from build123d import *

# Parameters (mm, degrees)
SKETCH1_R           = 12.5
SKETCH1_R_2         = 9.5
BOSS_EXTRUDE1_DEPTH = 14
SKETCH2_W           = 64.506168934
SKETCH2_H           = 47.83380527
BOSS_EXTRUDE2_DEPTH = 5
SKETCH3_R           = 7.5
CUT_EXTRUDE1_DEPTH  = 5
FILLET1_R           = 10
SKETCH4_R           = 41.339159207
SKETCH4_R_2         = 22.478966411
CUT_EXTRUDE2_DEPTH  = 10
SKETCH5_W           = 60
SKETCH5_H           = 44.957932822
SKETCH5_R           = 6
BOSS_EXTRUDE3_DEPTH = 5
FILLET2_R           = 5
SKETCH6_R           = 7.5
CUT_EXTRUDE3_DEPTH  = 10.435721216
SKETCH7_R           = 14
SKETCH7_R_2         = 12.5
BOSS_EXTRUDE4_DEPTH = 3.5
SKETCH8_R           = 13.175914581
SKETCH8_R_2         = 11.95
CUT_EXTRUDE4_DEPTH  = 2.5
BOSS_EXTRUDE5_START = -14
SKETCH9_R           = 9.5
SKETCH9_R_2         = 7.5
BOSS_EXTRUDE5_DEPTH = 14
SKETCH11_R          = 1.75
CUT_EXTRUDE5_DEPTH  = 6.2


with BuildPart() as part:
    # Sketch1 → Boss-Extrude1 (new body)
    with BuildSketch(Plane(origin=(0, 0, 0), x_dir=(1, 0, 0), z_dir=(0, 1, 0))):
        with Locations(Location((0, 0, 0), (0, 0, 270))):
            Circle(SKETCH1_R)
        with Locations(Location((0, 0, 0), (0, 0, 270))):
            Circle(SKETCH1_R_2, mode=Mode.SUBTRACT)
    extrude(amount=BOSS_EXTRUDE1_DEPTH)

    # Sketch2 → Boss-Extrude2 (add)
    with BuildSketch(Plane(origin=(0, 0, 0), x_dir=(-1, 0, 0), z_dir=(0, -1, 0))):
        Rectangle(SKETCH2_W, SKETCH2_H)
    extrude(amount=BOSS_EXTRUDE2_DEPTH)

    # Sketch3 → Cut-Extrude1 (cut)
    with BuildSketch(Plane(origin=(0, 0, 0), x_dir=(1, 0, 0), z_dir=(0, 1, 0))):
        with Locations(Location((0, 0, 0), (0, 0, 270))):
            Circle(SKETCH3_R)
    extrude(amount=-CUT_EXTRUDE1_DEPTH, mode=Mode.SUBTRACT)

    # Fillet1
    fillet1_edges = [part.edges().sort_by_distance(p)[0] for p in [
        (32.253084467, -2.5, -23.916902635),
        (32.253084467, -2.5, 23.916902635),
        (-32.253084467, -2.5, 23.916902635),
        (-32.253084467, -2.5, -23.916902635),
    ]]
    fillet(fillet1_edges, radius=FILLET1_R)

    # Sketch4 → Cut-Extrude2 (cut)
    with BuildSketch(Plane(origin=(0, 0, 0), x_dir=(1, 0, 0), z_dir=(0, 1, 0))):
        Circle(SKETCH4_R)
        with Locations(Location((0, 0, 0), (0, 0, 270))):
            Circle(SKETCH4_R_2, mode=Mode.SUBTRACT)
    extrude(amount=-CUT_EXTRUDE2_DEPTH, mode=Mode.SUBTRACT)

    # Sketch5 → Boss-Extrude3 (add)
    with BuildSketch(Plane(origin=(0, -5, 0), x_dir=(-1, 0, 0), z_dir=(0, -1, 0))):
        Rectangle(SKETCH5_W, SKETCH5_H)
        with Locations(Location((0, 0, 0), (0, 0, 90))):
            Circle(SKETCH5_R, mode=Mode.SUBTRACT)
    extrude(amount=-BOSS_EXTRUDE3_DEPTH)

    # Fillet2
    fillet2_edges = [part.edges().sort_by_distance(p)[0] for p in [
        (30, -2.5, -22.478966411),
        (-30, -2.5, 22.478966411),
        (30, -2.5, 22.478966411),
        (-30, -2.5, -22.478966411),
    ]]
    fillet(fillet2_edges, radius=FILLET2_R)

    # Sketch6 → Cut-Extrude3 (cut)
    with BuildSketch(Plane(origin=(0, -5, 0), x_dir=(-1, 0, 0), z_dir=(0, -1, 0))):
        with Locations(Location((0, 0, 0), (0, 0, 90))):
            Circle(SKETCH6_R)
    extrude(amount=-CUT_EXTRUDE3_DEPTH, mode=Mode.SUBTRACT)

    # Sketch7 → Boss-Extrude4 (add)
    with BuildSketch(Plane(origin=(0, 0, 0), x_dir=(1, 0, 0), z_dir=(0, 1, 0))):
        with Locations(Location((0, 0, 0), (0, 0, 270))):
            Circle(SKETCH7_R)
        with Locations(Location((0, 0, 0), (0, 0, 270))):
            Circle(SKETCH7_R_2, mode=Mode.SUBTRACT)
    extrude(amount=BOSS_EXTRUDE4_DEPTH)

    # Sketch8 → Cut-Extrude4 (cut)
    with BuildSketch(Plane(origin=(0, 13, 0), x_dir=(1, 0, 0), z_dir=(0, 1, 0))):
        Circle(SKETCH8_R)
        with Locations(Location((0, 0, 0), (0, 0, 270))):
            Circle(SKETCH8_R_2, mode=Mode.SUBTRACT)
    extrude(amount=-CUT_EXTRUDE4_DEPTH, mode=Mode.SUBTRACT)

    # Sketch9 → Boss-Extrude5 (add)
    with BuildSketch(Plane(origin=(0, 14, 0), x_dir=(1, 0, 0), z_dir=(0, 1, 0)).offset(BOSS_EXTRUDE5_START)):
        Circle(SKETCH9_R)
        with Locations(Location((0, 0, 0), (0, 0, 90))):
            Circle(SKETCH9_R_2, mode=Mode.SUBTRACT)
    extrude(amount=BOSS_EXTRUDE5_DEPTH)

    # Sketch11 → Cut-Extrude5 (cut)
    with BuildSketch(Plane(origin=(0, 0, 0), x_dir=(1, 0, 0), z_dir=(0, 1, 0))):
        with Locations(Location((-25, 17.478966411, 0), (0, 0, 270))):
            Circle(SKETCH11_R)
        with Locations(Location((25, 17.478966411, 0), (0, 0, 270))):
            Circle(SKETCH11_R)
        with Locations(Location((25, -17.478966411, 0), (0, 0, 270))):
            Circle(SKETCH11_R)
        with Locations(Location((-25, -17.478966411, 0), (0, 0, 270))):
            Circle(SKETCH11_R)
    extrude(amount=-CUT_EXTRUDE5_DEPTH, mode=Mode.SUBTRACT)


solid = part.part
Design review of the part built by this model. Coordinates are the model's own, in mm. A direction names the side the tool comes from. Round coordinates to 2 decimals unless told otherwise and drop trailing zeros. Loops run counter-clockwise (first coordinate to the right, second up) from the corner with the lowest first, then second, coordinate; pieces in that order, holes last. Notation, with made-up numbers: (27.5, -39) - (64.5, -39) arc R17 ccw to (64.5, -22) - close; hole circle Ø3 at (79.25, -35.5). An arc over 180 degrees is marked (long way). One line per question, with ' | ' between items.
1. We need section A-A, the plane x = 0. State the section outline as (y, z) points, and give its area (3 significant figures).
Results are:
outline: (-5, -22.48) - (0, -22.48) - (0, -14) - (3.5, -14) - (3.5, -12.5) - (10.5, -12.5) - (10.5, -11.95) - (13, -11.95) - (13, -12.5) - (14, -12.5) - (14, -7.5) - (-5, -7.5) - close; (-5, 7.5) - (14, 7.5) - (14, 12.5) - (13, 12.5) - (13, 11.95) - (10.5, 11.95) - (10.5, 12.5) - (3.5, 12.5) - (3.5, 14) - (0, 14) - (0, 22.48) - (-5, 22.48) - close | area: 298 mm²
2. Clearance check with flat-ended pins moving along their axes: P1, Ø3, axis at y = 8.5, z = 6, coming from the +X side; P2, Ø2, axis at x = 25, z = -17.48, coming from the -Y side; P3, Ø8, axis at x = -22.5, z = 10, coming from the +Y side; P4, Ø8, axis at x = 9.5, y = 11.5, coming from the +Z side. State where each tip first meets the part, or that it passes through.
Results are:
P1: stops at x = 11.66 | P2: passes through | P3: stops at y = 0 | P4: stops at z = 11.16
3. We need section C-C, the plane y = -2.5. State the section outline as (x, z) points.
Results are:
outline: (-30, -17.48) arc R5 ccw to (-25, -22.48) - (25, -22.48) arc R5 ccw to (30, -17.48) - (30, 17.48) arc R5 ccw to (25, 22.48) - (-25, 22.48) arc R5 ccw to (-30, 17.48) - close; hole circle Ø3.5 at (-25, -17.48); hole circle Ø3.5 at (-25, 17.48); hole circle Ø15 at (0, 0); hole circle Ø3.5 at (25, -17.48); hole circle Ø3.5 at (25, 17.48)
4. We need section B-B, the plane z = 0. State the section outline as (x, y) points, and give its area (3 significant figures).
Results are:
outline: (-30, -5) - (-7.5, -5) - (-7.5, 14) - (-12.5, 14) - (-12.5, 13) - (-11.95, 13) - (-11.95, 10.5) - (-12.5, 10.5) - (-12.5, 3.5) - (-14, 3.5) - (-14, 0) - (-30, 0) - close; (7.5, -5) - (30, -5) - (30, 0) - (14, 0) - (14, 3.5) - (12.5, 3.5) - (12.5, 10.5) - (11.95, 10.5) - (11.95, 13) - (12.5, 13) - (12.5, 14) - (7.5, 14) - close | area: 373 mm²
5. For faces 1 (the face through (-30, -3, 0)), 2 (the face through (3.755, 6.951, 11.923)), list the 3-axis set-ups (+Z, -Z, +X, -X, +Y, -Y) from which the entire face can be reached by the end or side of a thin tool; tool diameter is ignored.
Results are:
face 1: +Z, -Z, -X, +Y, -Y | face 2: +Y
6. We need section D-D, the plane y = 6.25. State the section outline as (x, z) points, and give its area (3 significant figures).
Results are:
outline: circle Ø25 at (0, 0); hole circle Ø15 at (0, 0) | area: 314 mm²
7. For L1, parallel to Y at x = 24.5, z = 10; L2, parallel to X at y = 6.5, z = -2; L3, parallel to Z at x = -5.5, y = 9, list the stretches that pass through material, from the lowest coordinate up. Write a range as [from, to].
Results are:
L1: y = [-5, 0] | L2: x = [-12.34, -7.23], [7.23, 12.34] | L3: z = [-11.22, -5.1], [5.1, 11.22]
